Part print with two shaded views. Sizes in mm from the minimum x, y, z corner. Give positions to 0.01 mm unless a question says otherwise; leave off trailing zeros. Write each loop counter-clockwise with the first axis right and the second up, starting at its lowest first coordinate (ties: lowest second). Pieces come first, ordered by that corner, then holes. Notation, with made-up numbers: (47, -7.75) -> (65, -7.75) arc R18 cw to (65, 27.25) -> close; hole circle Ø3 at (-14, -35). An arc over 180 degrees is marked (long way). Answer in a Markdown table with one row per item. Add a question column.
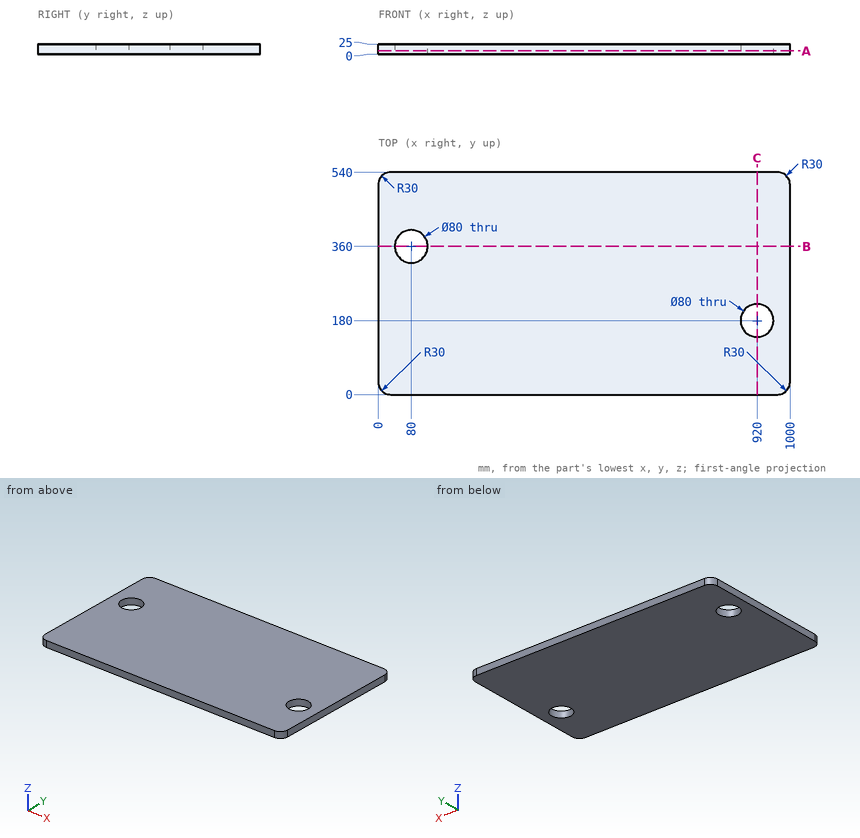
Item 1: Slice it at A-A, the plane z = 8. List the corners of the cut face in (x, y).
Item 2: Slice it at B-B, the plane y = 360. List the corners of the cut face in (x, z), then the cut area to 3 significant figures.
Item 3: Slice it at C-C, the plane x = 920. List the corners of the cut face in (y, z).
Item 4: Probe L1, parallel to Y at x = 920, z = 5.75; L2, parallel to Y at x = 80, z = 18; L3, parallel to X at y = 185.5, z = 1.75. List the from-to ranges inside material, lowest first. Write a range as from..to.
Answer key:
| question | item | result |
|---|---|---|
| 1 | outline | (0, 30) arc R30 ccw to (30, 0) -> (970, 0) arc R30 ccw to (1000, 30) -> (1000, 510) arc R30 ccw to (970, 540) -> (30, 540) arc R30 ccw to (0, 510) -> close; hole circle Ø80 at (80, 360); hole circle Ø80 at (920, 180) |
| 2 | outline | (0, 0) -> (40, 0) -> (40, 25) -> (0, 25) -> close; (120, 0) -> (1000, 0) -> (1000, 25) -> (120, 25) -> close |
| 2 | area | 23,000 mm² |
| 3 | outline | (0, 0) -> (140, 0) -> (140, 25) -> (0, 25) -> close; (220, 0) -> (540, 0) -> (540, 25) -> (220, 25) -> close |
| 4 | L1 | y = 0..140, 220..540 |
| 4 | L2 | y = 0..320, 400..540 |
| 4 | L3 | x = 0..880.38, 959.62..1000 |
